from build123d import *

# Parameters (mm, degrees)
BOSS_EXTRUDE1_DEPTH  = 5
SKETCH8_W            = 12.7
SKETCH8_H            = 25.4
CUT_EXTRUDE1_DEPTH   = 12.7
BOSS_EXTRUDE6_START  = 1.27
BOSS_EXTRUDE6_DEPTH  = 22.86
FILLET3_R            = 2.54
SKETCH12_W           = 22.86
SKETCH12_H           = 5.08
BOSS_EXTRUDE7_DEPTH  = 5.08
FILLET8_R            = 2.54
SKETCH13_W           = 2.54
SKETCH13_H           = 17.78
CUT_EXTRUDE2_DEPTH   = 2.032
BOSS_EXTRUDE8_DEPTH  = 22.86
FILLET5_R            = 2.54
FILLET6_R            = 2.54
BOSS_EXTRUDE9_START  = -27.94
SKETCH15_W           = 10.16
SKETCH15_H           = 3.81
BOSS_EXTRUDE9_DEPTH  = 12.7
BOSS_EXTRUDE10_START = -116.84
SKETCH15_2_W         = 10.16
SKETCH15_2_H         = 3.81
BOSS_EXTRUDE10_DEPTH = 12.7
FILLET7_R            = 2.54


with BuildPart() as part:
    # Sketch2 → Boss-Extrude1 (new body)
    with BuildSketch(Plane(origin=(0, 0, 0), x_dir=(1, 0, 0), z_dir=(0, 1, 0))):
        with BuildLine():
            Line((-98.109845206, -87.510053172), (50.472154842, -87.510053172))
            ThreePointArc((50.472154842, -87.510053172), (54.064257291, -86.02215562), (55.552154842, -82.430053172))
            Line((55.552154842, -82.430053172), (55.552154842, 66.389946828))
            ThreePointArc((55.552154842, 66.389946828), (54.064257291, 69.982049277), (50.472154842, 71.469946828))
            Line((50.472154842, 71.469946828), (-98.109845206, 71.469946828))
            ThreePointArc((-98.109845206, 71.469946828), (-101.701947654, 69.982049277), (-103.189845206, 66.389946828))
            Line((-103.189845206, 66.389946828), (-103.189845206, -82.430053172))
            ThreePointArc((-103.189845206, -82.430053172), (-101.701947654, -86.02215562), (-98.109845206, -87.510053172))
        make_face()
    extrude(amount=BOSS_EXTRUDE1_DEPTH)

    # Sketch8 → Cut-Extrude1 (cut)
    with BuildSketch(Plane(origin=(0, 5, 0), x_dir=(1, 0, 0), z_dir=(0, 1, 0))):
        with Locations((-96.839845206, -7.270053172)):
            Rectangle(SKETCH8_W, SKETCH8_H)
    extrude(amount=-CUT_EXTRUDE1_DEPTH, mode=Mode.SUBTRACT)

    # Sketch9 → Boss-Extrude6 (add)
    with BuildSketch(Plane(origin=(0, 0, 19.970053172), x_dir=(-1, 0, 0), z_dir=(0, 0, -1)).offset(BOSS_EXTRUDE6_START)):
        with BuildLine():
            Line((90.489845206, 5), (90.489845206, -9.510091846))
            ThreePointArc((90.489845206, -9.510091846), (91.233793982, -11.30614307), (93.029845206, -12.050091846))
            Line((93.029845206, -12.050091846), (100.984663509, -12.050091846))
            ThreePointArc((100.984663509, -12.050091846), (102.780714734, -11.30614307), (103.524663509, -9.510091846))
            Line((103.524663509, -9.510091846), (103.524663509, 5))
            Line((103.524663509, 5), (100.984663509, 5))
            Line((100.984663509, 5), (100.984663509, -6.970091846))
            ThreePointArc((100.984663509, -6.970091846), (100.240714734, -8.76614307), (98.444663509, -9.510091846))
            Line((98.444663509, -9.510091846), (95.569845206, -9.510091846))
            ThreePointArc((95.569845206, -9.510091846), (93.773793982, -8.76614307), (93.029845206, -6.970091846))
            Line((93.029845206, -6.970091846), (93.029845206, 5))
            Line((93.029845206, 5), (90.489845206, 5))
        make_face()
    extrude(amount=BOSS_EXTRUDE6_DEPTH)

    # Fillet3
    fillet3_edges = [part.edges().sort_by_distance(p)[0] for p in [
        (-90.489845206, 0, 7.270053172),
    ]]
    fillet(fillet3_edges, radius=FILLET3_R)

    # Sketch12 → Boss-Extrude7 (add)
    with BuildSketch(Plane.ZY.offset(103.524663509)):
        with Locations((7.270053172, 2.46)):
            Rectangle(SKETCH12_W, SKETCH12_H)
    extrude(amount=BOSS_EXTRUDE7_DEPTH)

    # Fillet8
    fillet8_edges = [part.edges().sort_by_distance(p)[0] for p in [
        (-100.984663509, 5, 7.270053172),
    ]]
    fillet(fillet8_edges, radius=FILLET8_R)

    # Sketch13 → Cut-Extrude2 (cut)
    with BuildSketch(Plane(origin=(0, 5, 0), x_dir=(1, 0, 0), z_dir=(0, 1, 0))):
        with Locations((-106.064663509, -7.270053172)):
            Rectangle(SKETCH13_W, SKETCH13_H)
    extrude(amount=-CUT_EXTRUDE2_DEPTH, mode=Mode.SUBTRACT)

    # Sketch14 → Boss-Extrude8 (add)
    with BuildSketch(Plane(origin=(0, 0, -4.159946828), x_dir=(-1, 0, 0), z_dir=(0, 0, -1))):
        Polygon((103.524663509, -4.576775108), (105.048663509, -4.576775108), (103.524663509, -7.370775108), align=None)
    extrude(amount=-BOSS_EXTRUDE8_DEPTH)

    # Fillet5
    fillet5_edges = [part.edges().sort_by_distance(p)[0] for p in [
        (-93.029845206, 5, 7.270053172),
    ]]
    fillet(fillet5_edges, radius=FILLET5_R)

    # Fillet6
    fillet6_edges = [part.edges().sort_by_distance(p)[0] for p in [
        (-108.604663509, -0.08, 7.270053172),
    ]]
    fillet(fillet6_edges, radius=FILLET6_R)

    # Sketch15 → Boss-Extrude9 (add)
    with BuildSketch(Plane(origin=(0, 0, -71.469946828), x_dir=(-1, 0, 0), z_dir=(0, 0, -1)).offset(BOSS_EXTRUDE9_START)):
        with Locations((-54.290154794, -1.905)):
            Rectangle(SKETCH15_W, SKETCH15_H)
    extrude(amount=-BOSS_EXTRUDE9_DEPTH)

    # Sketch15<2> → Boss-Extrude10 (add)
    with BuildSketch(Plane(origin=(0, 0, -71.469946828), x_dir=(-1, 0, 0), z_dir=(0, 0, -1)).offset(BOSS_EXTRUDE10_START)):
        with Locations((-54.290154794, -1.905)):
            Rectangle(SKETCH15_2_W, SKETCH15_2_H)
    extrude(amount=-BOSS_EXTRUDE10_DEPTH)

    # Fillet7
    # the kernel refuses this fillet: 2.54 mm, written as the material it adds along each edge
    with BuildSketch(Plane(origin=(49.210154794, 0, 45.370053172), x_dir=(-1, 0, 0), z_dir=(0, 0, 1)), Plane(origin=(49.210154794, 0, -43.529946828), x_dir=(-1, 0, 0), z_dir=(0, 0, 1))) as fillet7_piece_1:
        with BuildLine():
            CenterArc((FILLET7_R, FILLET7_R), FILLET7_R, 180, 90)
            Line((0, FILLET7_R), (0, 0))
            Line((0, 0), (FILLET7_R, 0))
        make_face()
    extrude(amount=12.7)
    # the kernel refuses this fillet: 2.54 mm, written as the material it takes off along each edge
    with BuildSketch(Plane(origin=(59.370154794, 0, 39.020053172), x_dir=(-1, 0, 0), z_dir=(0, 0, 1)), Plane(origin=(59.370154794, -3.81, 39.020053172), x_dir=(0, 1, 0), z_dir=(0, 0, 1)), Plane(origin=(59.370154794, -3.81, -49.879946828), x_dir=(0, 1, 0), z_dir=(0, 0, 1)), Plane(origin=(59.370154794, 0, -49.879946828), x_dir=(-1, 0, 0), z_dir=(0, 0, 1))) as fillet7_2_piece_1:
        with BuildLine():
            CenterArc((FILLET7_R, FILLET7_R), FILLET7_R, 180, 90)
            Line((0, FILLET7_R), (0, 0))
            Line((0, 0), (FILLET7_R, 0))
        make_face()
    extrude(amount=25.4, mode=Mode.SUBTRACT)


solid = part.part
Geometry: final body of the model. Coordinates: model frame, mm. A direction names the side the tool comes from. Round coordinates to 2 decimals unless told otherwise and drop trailing zeros. Order: outer loops, then holes, each group sorted by start corner. A loop starts at its lowest first (then second) coordinate and runs counter-clockwise, first axis right, second up. Notation, with made-up numbers: (-9.5, -36.75) -> (17.5, -36.75) arc R19 cw to (17.5, -17.75) -> close; hole circle Ø11 at (68, -27). An arc over 180 degrees is marked (long way). Put each result on its own line as item: value. Start each with the question number.
Q1. Section A-A on z = 49. Return the cut outline in (x, y) (1 decimal), and give its area (3 significant figures).
Q2. Section B-B on x = -70. Return the cut outline in (y, z).
Q3. Line query: probe 1 along Y at (x, z) = (-55.5, -34.5); probe 2 along X at (y, z) = (-1.5, -4); probe 3 along X at (y, z) = (1, 27). Output: solid intervals per line, ascending.
Q4. Reachability of faces 4 (the flat face through (-103.525, -2, 7)), 5 (the flat face through (-103.19, 2, 51)), 6 (the flat face through (-93.03, -2, 7)), 7 (the flat face through (-97, 3, 19.97)) from +Z, -Z, +X, -X, +Y, -Y: full face, straight path, thin tool, end or side. Return the list, or none.
Q5. Pull-direction query (X, two-part tool) for faces 1 (the flat face through (-100.985, -2, 7)), 2 (the cylindrical face through (-101.662, 2.465, -70.021)), 3 (the flat face through (54, -2, -30.83)); classes: +X half, -X half, draft (parallel to the pull), parting line (faces both ways), or undercut.
Q6. First-contact query: pin 1 (5 mm diameter, centred on x = -1, z = -31, fed in from -Y); pin 2 (10 mm diameter, centred on x = 32, y = -9, fed in from +Z); pin 3 (1.6 mm diameter, centred on x = -105.5, y = 4, fed in from -Z); pin 4 (0.6 mm diameter, centred on y = -8, z = 10.5, fed in from -X). Flat tips, straight axial feed; report the tip coordinate or a pass-through.
Q7. Section C-C on z = 23.5. Return the cut outline in (x, y), and give its area (3 significant figures).
Ans:
1. outline: (-103.2, 0) -> (46.7, 0) arc R2.5 cw to (49.2, -2.5) -> (49.2, -3.8) -> (56.8, -3.8) arc R2.5 ccw to (59.3, -1.9) arc R2.5 ccw to (56.8, 0) -> (55.6, 0) -> (55.6, 5) -> (-103.2, 5) -> close
1. area: 831 mm2
2. outline: (0, -71.47) -> (5, -71.47) -> (5, 87.51) -> (0, 87.51) -> close
3. probe 1: y = 0 to 5
3. probe 2: x = -103.52 to -100.98, -93.03 to -90.27
3. probe 3: x = -103.19 to 55.55
4. face 4: +Z, -Z, -X
4. face 5: +Z, -X, +Y, -Y
4. face 6: +Y
4. face 7: -X, +Y, -Y
5. face 1: undercut
5. face 2: -X half
5. face 3: draft
6. pin 1: stops at y = 0
6. pin 2: passes through
6. pin 3: stops at z = -4.16
6. pin 4: stops at x = -103.52
7. outline: (-103.19, 0) -> (55.55, 0) -> (55.55, 5) -> (-103.19, 5) -> close
7. area: 794 mm2
